Build history of the part. All positions in model axes, mm. A direction names the side the tool comes from. Give positions to 0.01 mm unless a question says otherwise; leave off trailing zeros. Order: outer loops, then holes, each group sorted by start corner. A loop starts at its lowest first (then second) coordinate and runs counter-clockwise, first axis right, second up. Notation, with made-up numbers: (82.5, 10) -> (140.5, 10) arc R27 cw to (140.5, 27) -> close; hole circle Ø6 at (21.5, -22.75). An arc over 180 degrees is marked (long way). One line per item, written item: value. Start each with the question number.
(1) Which spindle directions (+Z, -Z, +X, -X, +Y, -Y) get a long thin tool onto all of the face, cutting with end or side? Do faces 1 (the flat face through (1.5, -12, 25)), 2 (the flat face through (0, -29.217, 25)). Say none if no direction does.
(2) Saw through at D-D on z = 21. Give the cut face in (x, y).
(3) Saw through at B-B on y = -25.25. Give the cut face in (x, z).
(4) Two-plate mould, pull along X, no slides. Class faces 3 (the flat face through (1.77, -12.52, 16.02)), 4 (the cylindrical face through (-6.074, -27.713, 24.649)), 5 (the cylindrical face through (6.56, -12.3, 24.98)), 6 (the flat face through (0, -13.485, 25)): +X half, -X half, draft (parallel to the pull), parting line (faces both ways), or undercut.
(5) Saw through at A-A on x = 5. Give the cut face in (y, z).
(6) Probe line 1 (Y direction, x = 0.25, z = 18.75); line 2 (X direction, y = -22.25, z = 31.75); line 3 (X direction, y = -25.25, z = 26.25). List the from-to ranges inside material, lowest first.
(7) Saw through at C-C on z = 35.25. Give the cut face in (x, y).
(8) Pin check, flat tips, straight feed: pin 1 (1 mm diameter, centred on y = -12, z = 28, fed in from +X); pin 2 (2 mm diameter, centred on y = -12.5, z = 22.5, fed in from -X); pin 3 (2 mm diameter, centred on x = 3.5, y = -12.5, fed in from +Z). Stop position of each tip, or through.
```python
from build123d import *

# Parameters (mm, degrees)
BOSS_EXTRUDE1_DEPTH = 7.5
FILLET3_R           = 5
SKETCH4_R           = 2
SKETCH4_W           = 3
SKETCH4_H           = 2
CUT_EXTRUDE1_DEPTH  = 100
FILLET4_R           = 5
FILLET5_R           = 5


with BuildPart() as part:
    # Sketch1 → Boss-Extrude1 (new, symmetric)
    with BuildSketch(Plane(origin=(0, 0, 0), x_dir=(0, 0, -1), z_dir=(1, 0, 0))):
        Polygon((-31.324369962, -10.21673477), (-37.324369962, -16.21673477), (-37.324369962, -29.21673477), (-12.324369962, -29.21673477), (-12.324369962, -16.21673477), (-18.324369962, -10.21673477), align=None)
    extrude(amount=BOSS_EXTRUDE1_DEPTH, both=True)

    # Fillet3
    fillet3_edges = [part.edges().sort_by_distance(p)[0] for p in [
        (0, -16.21673477, 12.324369962),
        (0, -16.21673477, 37.324369962),
    ]]
    fillet(fillet3_edges, radius=FILLET3_R)

    # Sketch4 → Cut-Extrude1 (cut, symmetric)
    with BuildSketch(Plane.XY):
        with Locations((-3.5, -23.752268676)):
            Circle(SKETCH4_R)
        with Locations((3.5, -23.752268676)):
            Circle(SKETCH4_R)
        with Locations((0, -12.484501723)):
            Rectangle(SKETCH4_W, SKETCH4_H)
    extrude(amount=CUT_EXTRUDE1_DEPTH, both=True, mode=Mode.SUBTRACT)

    # Fillet4
    fillet4_edges = [part.edges().sort_by_distance(p)[0] for p in [
        (7.5, -29.21673477, 24.824369962),
        (-7.5, -29.21673477, 24.824369962),
    ]]
    fillet(fillet4_edges, radius=FILLET4_R)

    # Fillet5
    fillet5_edges = [part.edges().sort_by_distance(p)[0] for p in [
        (7.5, -10.21673477, 24.824369962),
        (-7.5, -10.21673477, 24.824369962),
    ]]
    fillet(fillet5_edges, radius=FILLET5_R)


solid = part.part
```
Results below:
1. face 1: +Z, -Z
1. face 2: +Z, -Z, +X, -X, -Y
2. outline: (-7.5, -24.22) arc R5 ccw to (-2.5, -29.22) -> (2.5, -29.22) arc R5 ccw to (7.5, -24.22) -> (7.5, -15.22) arc R5 ccw to (2.5, -10.22) -> (-2.5, -10.22) arc R5 ccw to (-7.5, -15.22) -> close; hole circle Ø4 at (-3.5, -23.75); hole (-1.5, -13.48) -> (1.5, -13.48) -> (1.5, -11.48) -> (-1.5, -11.48) -> close; hole circle Ø4 at (3.5, -23.75)
3. outline: (-7.39, 12.32) -> (-4.83, 12.32) -> (-4.83, 37.32) -> (-7.39, 37.32) -> close; (-2.17, 12.32) -> (2.17, 12.32) -> (2.17, 37.32) -> (-2.17, 37.32) -> close; (4.83, 12.32) -> (7.39, 12.32) -> (7.39, 37.32) -> (4.83, 37.32) -> close
4. face 3: draft
4. face 4: -X half
4. face 5: +X half
4. face 6: undercut
5. outline: (-28.55, 12.32) -> (-25.08, 12.32) -> (-25.08, 37.32) -> (-28.55, 37.32) -> close; (-22.43, 12.32) -> (-18.29, 12.32) arc R5 ccw to (-14.75, 13.79) -> (-10.89, 17.65) -> (-10.89, 31.99) -> (-14.75, 35.86) arc R5 ccw to (-18.29, 37.32) -> (-22.43, 37.32) -> close
6. line 1: y = -29.22 to -13.48, -11.48 to -10.22
6. line 2: x = -7.5 to -4.82, -2.18 to 2.18, 4.82 to 7.5
6. line 3: x = -7.39 to -4.83, -2.17 to 2.17, 4.83 to 7.39
7. outline: (-7.5, -24.22) arc R5 ccw to (-2.5, -29.22) -> (2.5, -29.22) arc R5 ccw to (7.5, -24.22) -> (7.5, -15.22) arc R5 ccw to (7.38, -14.14) -> (-7.38, -14.14) arc R5 ccw to (-7.5, -15.22) -> close; hole circle Ø4 at (-3.5, -23.75); hole circle Ø4 at (3.5, -23.75)
8. pin 1: stops at x = 6.7
8. pin 2: stops at x = -7.2
8. pin 3: stops at z = 34.61
